Geometry: see drawing. Coordinates: mm, zero at the bounding-box minimum. Coordinates: 2 decimals unless noted, no trailing zeros. Write each loop counter-clockwise with the first axis right and the second up, starting at its lowest first coordinate (ties: lowest second). Pieces come first, ordered by that corner, then holes.
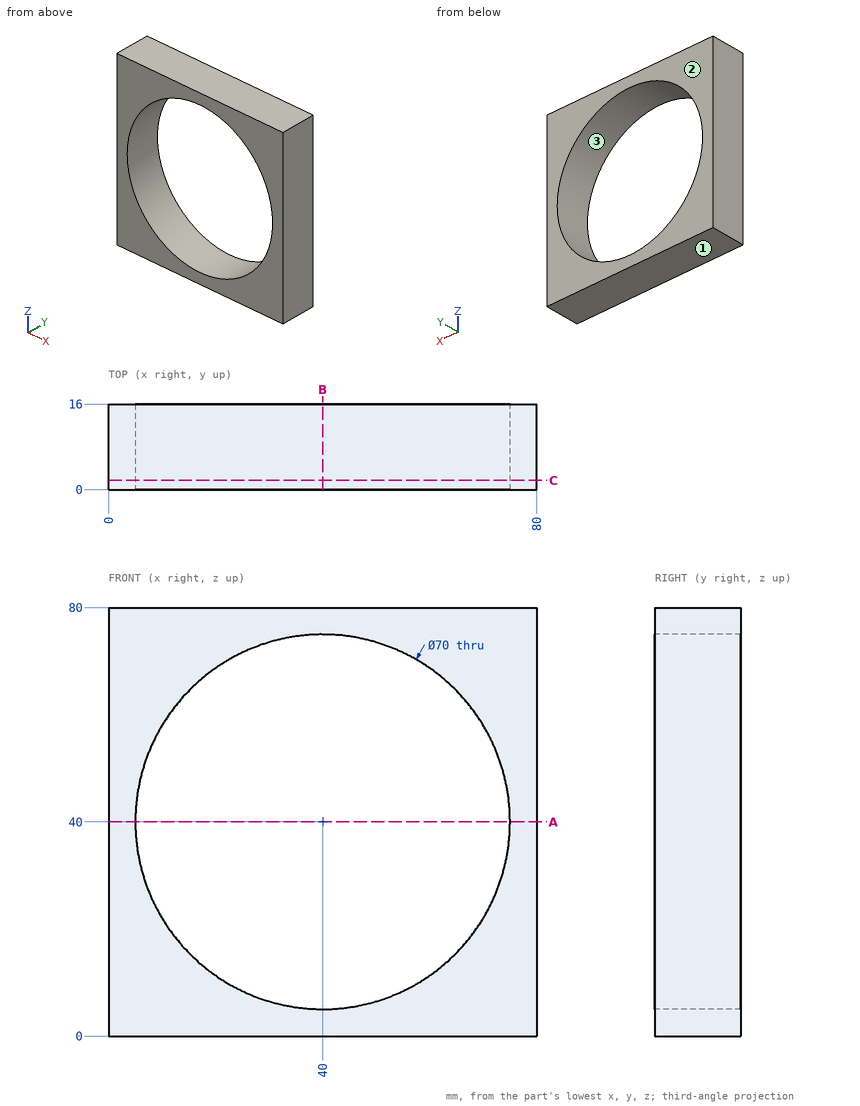
Item 1: Material intervals for probe 1 along Z at (x, y) = (40, 7.75); probe 2 along Z at (x, y) = (63.5, 8); probe 3 along X at (y, z) = (7.75, 25), sorted ascending.
Derived:
probe 1: z = 0 to 5, 75 to 80
probe 2: z = 0 to 14.06, 65.94 to 80
probe 3: x = 0 to 8.38, 71.62 to 80
Item 2: Section B-B, the plane x = 40. Output: boundary loops of the cut face in (y, z).
Derived:
outline: (0, 0) - (16, 0) - (16, 5) - (0, 5) - close; (0, 75) - (16, 75) - (16, 80) - (0, 80) - close
Item 3: Pin query (flat end, axial travel): pin 1 (6 mm diameter, centred on x = 18.5, z = 19, fed in from -Y). Return the tip coordinate at first contact, or that it passes through.
Derived:
pin 1: passes through
Item 4: Section C-C, the plane y = 1.75. Output: boundary loops of the cut face in (x, z), plus the area to 3 significant figures.
Derived:
outline: (0, 0) - (80, 0) - (80, 80) - (0, 80) - close; hole circle Ø70 at (40, 40)
area: 2,550 mm2
Item 5: Pull-direction query (Z, two-part tool) for the marked faces 1, 2 and 3; classes: released by +Z, released by -Z, zero draft, split by the parting line, or undercut.
Derived:
face 1: released by -Z
face 2: zero draft
face 3: undercut
Item 6: Section A-A, the plane z = 40. Output: boundary loops of the cut face in (x, y), plus the area to 3 significant figures.
Derived:
outline: (0, 0) - (5, 0) - (5, 16) - (0, 16) - close; (75, 0) - (80, 0) - (80, 16) - (75, 16) - close
area: 160 mm2
